Here's how the part is built. I have some questions about the finished solid (model axes, mm). Face numbers are marked on the shaded views. Give positions to 0.01 mm unless a question says otherwise; leave off trailing zeros. Write each loop counter-clockwise with the first axis right and the second up, starting at its lowest first coordinate (ties: lowest second). Pieces come first, ordered by that corner, then holes. Notation, with made-up numbers: (19.5, 9) - (74.5, 9) arc R13 ccw to (74.5, 13) - close; hole circle Ø7 at (67, 86.25). An arc over 180 degrees is marked (long way). Use a Markdown table: item, result.
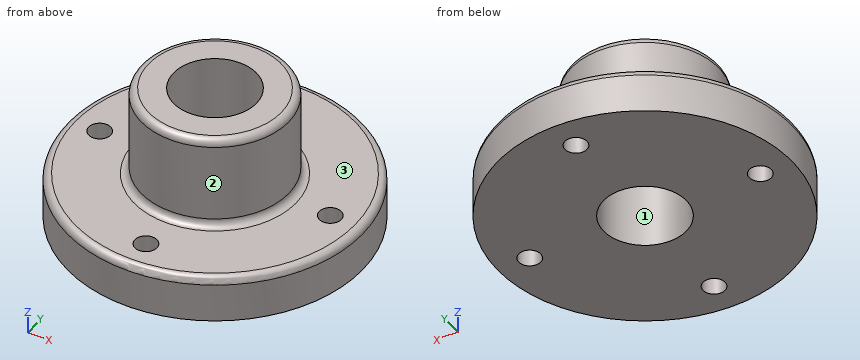
```python
from build123d import *

# Parameters (mm, degrees)
ESQUISSE1_R         = 80
BASE_25MM_DEPTH     = 25
ESQUISSE1_4_R       = 40
AXE75MM_DEPTH       = 75
TROU1_REACH         = 137.739
ESQUISSE1_5_R       = 6
TROU2_REACH         = 137.739
ESQUISSE1_6_R       = 6
TROU3_4_REACH       = 137.739
ESQUISSE1_7_R       = 6
TROUPRINCIPAL_REACH = 137.739
ESQUISSE1_8_R       = 22.5
CONG_1_R            = 4
CONG_2_R            = 4
CONG_3_R            = 4


with BuildPart() as part:
    # Esquisse1 → Base 25mm (new body)
    with BuildSketch(Plane.XY):
        Circle(ESQUISSE1_R)
    extrude(amount=BASE_25MM_DEPTH)

    # Esquisse1<4> → axe75mm (add)
    with BuildSketch(Plane.XY):
        Circle(ESQUISSE1_4_R)
    extrude(amount=AXE75MM_DEPTH)

    # Esquisse1<5> → Trou1 (cut, up to next)
    with BuildSketch(Plane.XY, mode=Mode.PRIVATE) as trou1_sk1:
        with Locations((0, 62.5)):
            Circle(ESQUISSE1_5_R)
    trou1_tool1 = extrude(trou1_sk1.sketch, amount=TROU1_REACH, mode=Mode.PRIVATE) & part.part
    add(trou1_tool1.solids().sort_by_distance((0, 62.5, 0))[0], mode=Mode.SUBTRACT)

    # Esquisse1<6> → Trou2 (cut, up to next)
    with BuildSketch(Plane.XY, mode=Mode.PRIVATE) as trou2_sk1:
        with Locations((-62.5, 0)):
            Circle(ESQUISSE1_6_R)
    trou2_tool1 = extrude(trou2_sk1.sketch, amount=TROU2_REACH, mode=Mode.PRIVATE) & part.part
    add(trou2_tool1.solids().sort_by_distance((-62.5, 0, 0))[0], mode=Mode.SUBTRACT)

    # Esquisse1<7> → Trou3&4 (cut, up to next)
    with BuildSketch(Plane.XY, mode=Mode.PRIVATE) as trou3_4_sk1:
        with Locations((62.5, 0)):
            Circle(ESQUISSE1_7_R)
    trou3_4_tool1 = extrude(trou3_4_sk1.sketch, amount=TROU3_4_REACH, mode=Mode.PRIVATE) & part.part
    # Esquisse1<7> → Trou3&4 (cut, up to next)
    with BuildSketch(Plane.XY, mode=Mode.PRIVATE) as trou3_4_sk2:
        with Locations((0, -62.5)):
            Circle(ESQUISSE1_7_R)
    trou3_4_tool2 = extrude(trou3_4_sk2.sketch, amount=TROU3_4_REACH, mode=Mode.PRIVATE) & part.part
    add(trou3_4_tool1.solids().sort_by_distance((62.5, 0, 0))[0], mode=Mode.SUBTRACT)
    add(trou3_4_tool2.solids().sort_by_distance((0, -62.5, 0))[0], mode=Mode.SUBTRACT)

    # Esquisse1<8> → TrouPrincipal (cut, up to next)
    with BuildSketch(Plane.XY, mode=Mode.PRIVATE) as trouprincipal_sk1:
        Circle(ESQUISSE1_8_R)
    trouprincipal_tool1 = extrude(trouprincipal_sk1.sketch, amount=TROUPRINCIPAL_REACH, mode=Mode.PRIVATE) & part.part
    add(trouprincipal_tool1.solids().sort_by_distance((0, 0, 0))[0], mode=Mode.SUBTRACT)

    # Congé1
    cong_1_edges = [part.edges().sort_by_distance(p)[0] for p in [
        (-40, 0, 25),
    ]]
    fillet(cong_1_edges, radius=CONG_1_R)

    # Congé2
    cong_2_edges = [part.edges().sort_by_distance(p)[0] for p in [
        (-80, 0, 25),
    ]]
    fillet(cong_2_edges, radius=CONG_2_R)

    # Congé3
    cong_3_edges = [part.edges().sort_by_distance(p)[0] for p in [
        (-40, 0, 75),
    ]]
    fillet(cong_3_edges, radius=CONG_3_R)


solid = part.part
```
Item 1: If we section it at D-D, the plane z = 44: Write out the boundary of the cut face in (x, y), plus the area to 3 significant figures.
Values:
| item | result |
|---|---|
| outline | circle Ø80 at (0, 0); hole circle Ø45 at (0, 0) |
| area | 3,440 mm2 |
Item 2: Thinking about a two-plate mould opening in Y: for the marked faces 1, 2 and 3, which applies, +Y half, -Y half, draft (parallel to the pull), parting line (faces both ways), or undercut?
Values:
| item | result |
|---|---|
| face 1 | undercut |
| face 2 | parting line |
| face 3 | draft |
Item 3: I need wall thicknesses on line 1 along Y through (x, z) = (-1, 47); line 2 along Z through (x, y) = (55, -49); line 3 along Y through (x, z) = (-19, 12). Which ranges of each line are inside material? Lowest first, please. Write a range as [from, to].
Values:
| item | result |
|---|---|
| line 1 | y = [-39.99, -22.48], [22.48, 39.99] |
| line 2 | z = [0, 25] |
| line 3 | y = [-77.71, -12.05], [12.05, 77.71] |
Item 4: Will these pins go through, and if not, where does the flat tip stop? pin 1 Ø4 at (x, y) = (28.5, 61) entering from -Z; pin 2 Ø8 at (y, z) = (-41.5, 24) entering from +X; pin 3 Ø1.5 at (x, z) = (34, 21.5) entering from -Y; pin 4 Ø2 at (y, z) = (-23, 39.5) entering from -X.
Values:
| item | result |
|---|---|
| pin 1 | stops at z = 0 |
| pin 2 | stops at x = 70.24 |
| pin 3 | stops at y = -72.74 |
| pin 4 | stops at x = -33.41 |
Item 5: If we section it at A-A, the plane y = 0: Write out the boundary of the cut face in (x, z), plus the area to 3 significant figures.
Values:
| item | result |
|---|---|
| outline | (-80, 0) - (-68.5, 0) - (-68.5, 25) - (-76, 25) arc R4 ccw to (-80, 21) - close; (-56.5, 0) - (-22.5, 0) - (-22.5, 75) - (-36, 75) arc R4 ccw to (-40, 71) - (-40, 29) arc R4 cw to (-44, 25) - (-56.5, 25) - close; (22.5, 0) - (56.5, 0) - (56.5, 25) - (44, 25) arc R4 cw to (40, 29) - (40, 71) arc R4 ccw to (36, 75) - (22.5, 75) - close; (68.5, 0) - (80, 0) - (80, 21) arc R4 ccw to (76, 25) - (68.5, 25) - close |
| area | 4,020 mm2 |
Item 6: If we section it at C-C, the plane z = 5: Write out the boundary of the cut face in (x, y), plus the area to 3 significant figures.
Values:
| item | result |
|---|---|
| outline | circle Ø160 at (0, 0); hole circle Ø12 at (-62.5, 0); hole circle Ø45 at (0, 0); hole circle Ø12 at (0, -62.5); hole circle Ø12 at (0, 62.5); hole circle Ø12 at (62.5, 0) |
| area | 18,100 mm2 |
